Could you check a few things on this model? Use its own coordinates, in mm. Face numbers are marked on the shaded views. A direction names the side the tool comes from. Give positions to 0.01 mm unless a question says otherwise; leave off trailing zeros. Loops run counter-clockwise (first coordinate to the right, second up) from the corner with the lowest first, then second, coordinate; pieces in that order, holes last. Notation, with made-up numbers: M -5,37.5 L 44,37.5 A26 ccw 44,72.5 Z; hole C -25.5,64 d9. An arc over 180 degrees is marked long. Write each question's results on one line, items separated by ' | '. Start each with the question number.
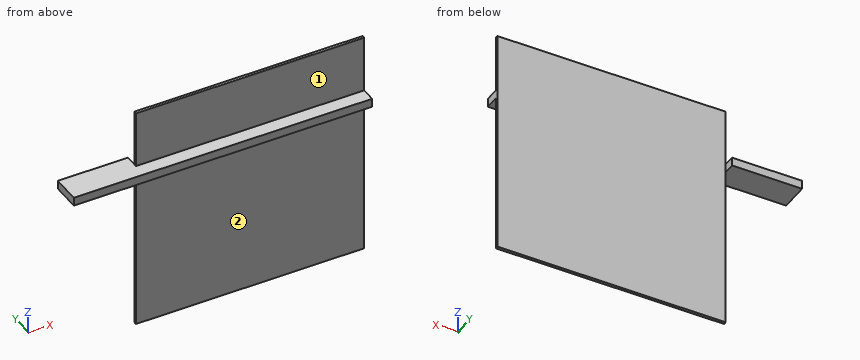
from build123d import *

# Parameters (mm, degrees)
BOSS_EXTRUDE3_DEPTH = 3
SKETCH4_W           = 80
SKETCH4_H           = 80
BOSS_EXTRUDE4_DEPTH = 1


with BuildPart() as part:
    # Sketch1 → Boss-Extrude3 (new body)
    with BuildSketch(Plane.XY):
        Polygon((15.553767031, 1.327814089), (15.553767031, 6.327814089), (-9.026232969, 6.327814089), (-9.026232969, -3.672185911), (5.238144653, -3.672185911), (95.553767031, -3.672185911), (95.553767031, 1.327814089), align=None)
    extrude(amount=BOSS_EXTRUDE3_DEPTH)

    # Sketch4 → Boss-Extrude4 (add)
    with BuildSketch(Plane(origin=(0, 1.327814089, 0), x_dir=(1, 0, 0), z_dir=(0, 1, 0))):
        with Locations((55.553767031, 17)):
            Rectangle(SKETCH4_W, SKETCH4_H)
    extrude(amount=BOSS_EXTRUDE4_DEPTH)


solid = part.part
1) If we section it at C-C on y = -0.5: Write out the boundary of the cut face in (x, z).
2) If we section it at B-B on z = 11: Write out the boundary of the cut face in (x, y).
3) If we section it at A-A on x = 22.5: Write out the boundary of the cut face in (y, z).
4) Please list where these lines run through material, in increasing order: line 1 (Z direction, x = 15, y = 2.5); line 2 (X direction, y = 1.75, z = 12.5); line 3 (Y direction, x = 25, z = -4.5). Write a range as from..to.
5) Which directions (+Z, -Z, +X, -X, +Y, -Y) give clear straight access to the entire face, cutting with the end or side of a thin tool? Please do the marked faces 1 and 2.
6) I'm going to push flat-ended pins straight in: P1, Ø8, axis at x = 46.5, z = 7.5, coming from the +Y side; P2, Ø5, axis at y = -1.5, z = -10, coming from the +X side; P3, Ø3, axis at x = 45.5, y = -2, coming from the -Z side; P4, Ø0.8, axis at y = 1.5, z = 11, coming from the -X side. Where does each tip first touch, or does it pass through?
Calculated:
1) outline: M -9.03,0 L 95.55,0 L 95.55,3 L -9.03,3 Z
2) outline: M 15.55,1.33 L 95.55,1.33 L 95.55,2.33 L 15.55,2.33 Z
3) outline: M -3.67,0 L 1.33,0 L 1.33,-57 L 2.33,-57 L 2.33,23 L 1.33,23 L 1.33,3 L -3.67,3 Z
4) line 1: z = 0..3 | line 2: x = 15.55..95.55 | line 3: y = 1.33..2.33
5) face 1: +Z, +X, -X, -Y | face 2: -Z, +X, -X, -Y
6) P1: stops at y = 2.33 | P2: passes through | P3: stops at z = 0 | P4: stops at x = 15.55
